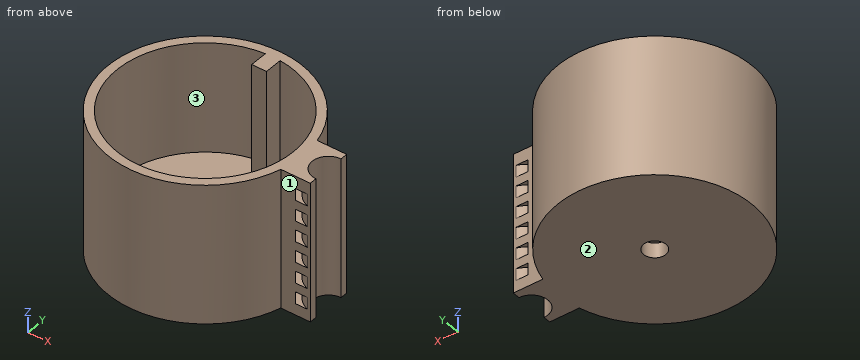
from build123d import *

# Parameters (mm, degrees)
F0_R           = 32.75
F1_DEPTH       = 40
F2_T           = -3
F3_DEPTH       = 7
F5_D           = 4.2
F5_DEPTH       = 15
F5_CBORE_D     = 7.5
F5_CBORE_DEPTH = 5
F5_TIP         = 1.2618073
F7_DEPTH       = 37
F9_DEPTH       = 47
F10_W          = 2
F10_H          = 4


with BuildPart() as f1:
    # F0 (on Top) → F1 (new body)
    with BuildSketch(Plane.XY):
        Circle(F0_R)
    extrude(amount=F1_DEPTH)

    # F2
    f2_openings = [f1.faces().sort_by_distance(p)[0] for p in [
        (0, 0, 40),
    ]]
    offset(amount=F2_T, openings=f2_openings)

    # F3 (add): a face of the model
    f3_faces = [f1.faces().sort_by_distance(p)[0] for p in [
        (0, 0, 0),
    ]]
    extrude(f3_faces, amount=F3_DEPTH)

    # F5
    with Locations(Plane(origin=(0, 0, -7), x_dir=(1, 0, 0), z_dir=(0, 0, -1))):
        with Locations((0, 0)):
            CounterBoreHole(F5_D / 2, F5_CBORE_D / 2, F5_CBORE_DEPTH, depth=F5_DEPTH)
            with Locations((0, 0, -(F5_DEPTH + F5_TIP / 2))):  # 118° drill point
                Cone(0, F5_D / 2, F5_TIP, mode=Mode.SUBTRACT)

    # F6 (on face) → F7 (join)
    with BuildSketch(Plane.XY.offset(3)):
        with BuildLine():
            ThreePointArc((2.5, 29.6447718831), (0, 29.75), (-2.5, 29.6447718831))
            Line((-2.5, 29.6447718831), (-2.5, 23.6447718831))
            Line((-2.5, 23.6447718831), (2.5, 23.6447718831))
            Line((2.5, 23.6447718831), (2.5, 29.6447718831))
        make_face()
    extrude(amount=F7_DEPTH)

    # F8 (on face) → F9 (join)
    with BuildSketch(Plane(origin=(0, 0, -7), x_dir=(1, 0, 0), z_dir=(0, 0, -1))):
        with BuildLine():
            ThreePointArc((32.75, 0), (32.5010218458, -4.0306425017), (31.7578730396, -8))
            Line((31.7578730396, -8), (41.7578730396, -8))
            Line((41.7578730396, -8), (41.7578730396, -5.5))
            ThreePointArc((41.7578730396, -5.5), (36.2578730396, 0), (41.7578730396, 5.5))
            Line((41.7578730396, 5.5), (41.7578730396, 8))
            Line((41.7578730396, 8), (31.7578730396, 8))
            ThreePointArc((31.7578730396, 8), (32.5010218458, 4.0306425017), (32.75, 0))
        make_face()
    extrude(amount=-F9_DEPTH)

    # F10 (on Front) → F11 (revolve, cut)
    with BuildSketch(Plane.XZ):
        with Locations((33.9883454144, -1.1719100263)):
            Rectangle(F10_W, F10_H)
        with Locations((33.9883454144, 5.8280899737)):
            Rectangle(F10_W, F10_H)
        with Locations((33.9883454144, 12.8280899737)):
            Rectangle(F10_W, F10_H)
        with Locations((33.9883454144, 19.8280899737)):
            Rectangle(F10_W, F10_H)
        with Locations((33.9883454144, 26.8280899737)):
            Rectangle(F10_W, F10_H)
        with Locations((33.9883454144, 33.8280899737)):
            Rectangle(F10_W, F10_H)
    revolve(axis=Axis((43.3594956994, 0, 17.8845692426), (0, 0, 1)), mode=Mode.SUBTRACT)


solid = f1.part
For this review, take the finished solid that the model builds, in its own axes (mm). Face numbers are marked on the shaded views. A direction names the side the tool comes from. Round coordinates to 2 decimals unless told otherwise and drop trailing zeros. Write each loop counter-clockwise with the first axis right and the second up, starting at its lowest first coordinate (ties: lowest second). Pieces come first, ordered by that corner, then holes. Notation, with made-up numbers: (57.25, -28.5) - (75.25, -28.5) arc R13 ccw to (75.25, -18.5) - close; hole circle Ø8 at (65, 17). An arc over 180 degrees is marked (long way). Write item = value, one per line. Start each with the question number.
1. Wall thickness on L1, parallel to Y at x = 0, z = 29.5; L2, parallel to X at y = 0, z = 17; L3, parallel to X at y = 0, z = 27: over which ranges is each line inside the solid? List them lowest first.
2. Consider section C-C on y = 0. Give the number of separate pieces and of enclosed holes in the cut face, plus the area to 3 significant figures.
3. Consider section A-A on x = 0. State the section outline as (y, z) points, plus the area to 3 significant figures.
4. Consider section B-B on z = -1. State the section outline as (x, y) points, plus the area to 3 significant figures.
5. Consider section D-D on y = -14. State the section outline as (x, z) points, plus the area to 3 significant figures.
6. For the marked faces 1, 2 and 3, list the 3-axis set-ups (+Z, -Z, +X, -X, +Y, -Y) from which the entire face can be reached by the end or side of a thin tool; tool diameter is ignored.
7. For pin 1 Ø3 at (y, z) = (17, 11.5) entering from -X; pin 2 Ø12 at (x, y) = (0, 0) entering from +Z; pin 3 Ø1 at (x, z) = (-6.5, 6.5) entering from +Y, all flat-tipped, find the tip position at first contact; note any pin that passes through.
Evaluation:
q1.L1 = -32.75 to -29.75, 23.64 to 32.75
q1.L2 = -32.75 to -29.75, 29.75 to 36.26
q1.L3 = -32.75 to -29.75, 29.75 to 32.99, 34.99 to 36.26
q2.separate_pieces = 2
q2.enclosed_holes = 6
q2.area = 935 mm2
q3.outline = (-32.75, -7) - (-3.75, -7) - (-3.75, -2) - (-2.1, -2) - (-2.1, 3) - (-29.75, 3) - (-29.75, 40) - (-32.75, 40) - close; (2.1, -2) - (3.75, -2) - (3.75, -7) - (32.75, -7) - (32.75, 40) - (23.64, 40) - (23.64, 3) - (2.1, 3) - close
q3.area = 1,040 mm2
q4.outline = (31.76, -8) - (36.76, -8) arc R10.37 cw to (36.76, 8) - (31.76, 8) arc R32.75 ccw (long way) to start; (40.89, -8) - (41.76, -8) - (41.76, -5.5) arc R5.5 cw to (41.76, 5.5) - (41.76, 8) - (40.89, 8) arc R8.37 ccw to start; hole circle Ø4.2 at (0, 0)
q4.area = 3,420 mm2
q5.outline = (-29.61, -7) - (29.61, -7) - (29.61, 40) - (26.25, 40) - (26.25, 3) - (-26.25, 3) - (-26.25, 40) - (-29.61, 40) - close
q5.area = 841 mm2
q6.face_1 = +Z, -Z, +X, -Y
q6.face_2 = -Z, +X, -X, +Y, -Y
q6.face_3 = +Z
q7.pin_1 = -28.85
q7.pin_2 = 3
q7.pin_3 = 32.2
